```python
from build123d import *

# Parameters (mm, degrees)
SM_BASE_FLANGE_1_DEPTH    = 37
CHAMFER_1_SIZE            = 2
HOLE_WIZARD_1_D           = 3.3
HOLE_WIZARD_1_DEPTH       = 3
HOLE_WIZARD_1_CBORE_D     = 5
HOLE_WIZARD_1_CBORE_DEPTH = 1
HOLE_WIZARD_1_TIP         = 0.991420021
HOLE_WIZARD_2_D           = 3.3
HOLE_WIZARD_2_DEPTH       = 3
HOLE_WIZARD_2_CBORE_D     = 5
HOLE_WIZARD_2_CBORE_DEPTH = 1
HOLE_WIZARD_2_TIP         = 0.991420021


# Sheet-metal steps are written as plain solids
with BuildPart() as part:
    # Sketch 1 → 基体-法兰1 (new body)
    with BuildSketch(Plane.XY):
        with BuildLine():
            Line((60.1, 7.55), (36.1, 7.55))
            ThreePointArc((36.1, 7.55), (33.978679656, 8.428679656), (33.1, 10.55))
            Line((33.1, 10.55), (33.1, 21.55))
            ThreePointArc((33.1, 21.55), (31.342640687, 25.792640687), (27.1, 27.55))
            Line((27.1, 27.55), (6, 27.55))
            ThreePointArc((6, 27.55), (1.757359313, 25.792640687), (0, 21.55))
            Line((0, 21.55), (0, 3))
            ThreePointArc((0, 3), (-0.878679656, 0.878679656), (-3, 0))
            Line((-3, 0), (-39, 0))
            Line((-39, 0), (-39, -3))
            Line((-39, -3), (-3, -3))
            ThreePointArc((-3, -3), (1.242640687, -1.242640687), (3, 3))
            Line((3, 3), (3, 21.55))
            ThreePointArc((3, 21.55), (3.878679656, 23.671320344), (6, 24.55))
            Line((6, 24.55), (27.1, 24.55))
            ThreePointArc((27.1, 24.55), (29.221320344, 23.671320344), (30.1, 21.55))
            Line((30.1, 21.55), (30.1, 10.55))
            ThreePointArc((30.1, 10.55), (31.857359313, 6.307359313), (36.1, 4.55))
            Line((36.1, 4.55), (60.1, 4.55))
            Line((60.1, 4.55), (60.1, 7.55))
        make_face()
    extrude(amount=SM_BASE_FLANGE_1_DEPTH)

    # 倒角1
    chamfer_1_edges = [part.edges().sort_by_distance(p)[0] for p in [
        (-39, -1.5, 0),
        (60.1, 6.05, 0),
        (-39, -1.5, 37),
        (60.1, 6.05, 37),
    ]]
    chamfer(chamfer_1_edges, length=CHAMFER_1_SIZE)

    # 打孔尺寸(%根据)内六角圆柱头螺钉的类型1
    with Locations(Plane(origin=(0, 7.55, 0), x_dir=(1, 0, 0), z_dir=(0, 1, 0))):
        with Locations((49.1, -6), (49.1, -31), (41.1, -31), (41.1, -6)):
            CounterBoreHole(HOLE_WIZARD_1_D / 2, HOLE_WIZARD_1_CBORE_D / 2, HOLE_WIZARD_1_CBORE_DEPTH, depth=HOLE_WIZARD_1_DEPTH)
            with Locations((0, 0, -(HOLE_WIZARD_1_DEPTH + HOLE_WIZARD_1_TIP / 2))):  # 118° drill point
                Cone(0, HOLE_WIZARD_1_D / 2, HOLE_WIZARD_1_TIP, mode=Mode.SUBTRACT)

    # 打孔尺寸(%根据)内六角圆柱头螺钉的类型2
    with Locations(Plane(origin=(0, 0, 0), x_dir=(1, 0, 0), z_dir=(0, 1, 0))):
        with Locations((-29, -8), (-9, -8), (-9, -29), (-29, -29)):
            CounterBoreHole(HOLE_WIZARD_2_D / 2, HOLE_WIZARD_2_CBORE_D / 2, HOLE_WIZARD_2_CBORE_DEPTH, depth=HOLE_WIZARD_2_DEPTH)
            with Locations((0, 0, -(HOLE_WIZARD_2_DEPTH + HOLE_WIZARD_2_TIP / 2))):  # 118° drill point
                Cone(0, HOLE_WIZARD_2_D / 2, HOLE_WIZARD_2_TIP, mode=Mode.SUBTRACT)


solid = part.part
```
Could you check a few things on this model? Use its own coordinates, in mm. A direction names the side the tool comes from. Round coordinates to 2 decimals unless told otherwise and drop trailing zeros. Loops run counter-clockwise (first coordinate to the right, second up) from the corner with the lowest first, then second, coordinate; pieces in that order, holes last.
Q1. For P1, Ø1.5, axis at x = 0, z = 28.5, coming from the +Y side; P2, Ø4, axis at x = 49.1, z = 6, coming from the -Y side; P3, Ø1.5, axis at y = 5.5, z = 10.5, coming from the -X side, each with a flat end and sliding along its axis, tell me the tip position at first contact or that it passes through.
Q2. Please list where these lines run through material, in increasing order: L1, parallel to Z at x = -29, y = -0.7; L2, parallel to Z at x = -9, y = -2; L3, parallel to X at y = 16, z = 23.
Q3. On a 3-axis mill with a long thin cutter (end or side, diameter ignored), from which of +Z, -Z, +X, -X, +Y, -Y can I reach the whole of each face in a straight line? I mean faces 1 (the cylindrical face through (29.2, 23.69, 18.24)), 2 (the cylindrical face through (42.75, 5.54, 5.93)), 3 (the flat face through (10, 25, 37)), 4 (the flat face through (48, 7.55, 18)), 5 (the flat face through (-27, -1, 9)). Say none if no direction works.
Q4. I want a section at C-C (z = 18). Write out the boundary of the cut face in (x, y).
Q5. I want a section at D-D (x = 34). Write out the boundary of the cut face in (y, z), and give its area (3 significant figures).
Q6. Thinking about a two-plate mould opening in Z: for faces 6 (the cylindrical face through (-9.33, -0.49, 26.52)), 7 (the flat face through (33.1, 16, 18)), 8 (the flat face through (59.1, 6, 1)), which applies, pulls with the +Z half, pulls with the -Z half, needs draft (parallel to the pull), parting line crosses it, or undercut?
Q7. I want a section at B-B (x = -29). Write out the boundary of the cut face in (y, z).
Q8. I want a section at A-A (y = 16). Write out the boundary of the cut face in (x, z), and give its area (3 significant figures).
Answer below:
1. P1: stops at y = 24.45
1. P2: stops at y = 4.55
1. P3: stops at x = 0
2. L1: z = 0 to 5.5, 10.5 to 26.5, 31.5 to 37
2. L2: z = 0 to 6.35, 9.65 to 27.35, 30.65 to 37
2. L3: x = 0 to 3, 30.1 to 33.1
3. face 1: +Z, -Z, -Y
3. face 2: +Y, -Y
3. face 3: +Z, +X, -X, +Y, -Y
3. face 4: +Z, -Z, +X, +Y
3. face 5: +Y
4. outline: (-39, -3) - (-3, -3) arc R6 ccw to (3, 3) - (3, 21.55) arc R3 cw to (6, 24.55) - (27.1, 24.55) arc R3 cw to (30.1, 21.55) - (30.1, 10.55) arc R6 ccw to (36.1, 4.55) - (60.1, 4.55) - (60.1, 7.55) - (36.1, 7.55) arc R3 cw to (33.1, 10.55) - (33.1, 21.55) arc R6 ccw to (27.1, 27.55) - (6, 27.55) arc R6 ccw to (0, 21.55) - (0, 3) arc R3 cw to (-3, 0) - (-39, 0) - close
5. outline: (4.93, 0) - (8.41, 0) - (8.41, 37) - (4.93, 37) - close
5. area: 129 mm2
6. face 6: undercut
6. face 7: needs draft
6. face 8: pulls with the -Z half
7. outline: (-3, 0) - (0, 0) - (0, 5.5) - (-1, 5.5) - (-1, 6.35) - (-3, 6.35) - close; (-3, 9.65) - (-1, 9.65) - (-1, 10.5) - (0, 10.5) - (0, 26.5) - (-1, 26.5) - (-1, 27.35) - (-3, 27.35) - close; (-3, 30.65) - (-1, 30.65) - (-1, 31.5) - (0, 31.5) - (0, 37) - (-3, 37) - close
8. outline: (0, 0) - (3, 0) - (3, 37) - (0, 37) - close; (30.1, 0) - (33.1, 0) - (33.1, 37) - (30.1, 37) - close
8. area: 222 mm2
